Verification items for this drawing (mm, ordinates from the low corner). A direction names the side the tool comes from. Round coordinates to 2 decimals unless told otherwise and drop trailing zeros. Order: outer loops, then holes, each group sorted by start corner. A loop starts at its lowest first (then second) coordinate and runs counter-clockwise, first axis right, second up. Notation, with made-up numbers: (-0.5, -8.75) - (7.5, -8.75) arc R14 cw to (7.5, 10.25) - close; hole circle Ø5 at (80.25, 18). An arc over 180 degrees is marked (long way). Use a Markdown table: item, result. Add a question column.
(1) Section check A-A on y = 4.85. Record the boundary of the cut face in (x, z), then the cut area to 3 significant figures.
(2) Section check D-D on y = 0.65. Record the boundary of the cut face in (x, z), then the cut area to 3 significant figures.
(3) Thickness scan on line 1 along Z through (x, y) = (6, 2.55); line 2 along Y through (x, z) = (4.5, 1). Record the ranges inside material, lowest first. Write a range as [from, to].
(4) Section check C-C on z = 1. Record the boundary of the cut face in (x, y).
(5) Section check B-B on x = 3.75. Record the boundary of the cut face in (y, z), then the cut area to 3 significant figures.
(6) Gauge pin test, flat ends, axial feed: P1, Ø1.6, axis at x = 4.5, z = 1.5, coming from the +Y side; P2, Ø1, axis at x = 3, y = 1.5, coming from the +Z side; P3, Ø1.6, axis at x = 1.5, y = 4.5, coming from the +Z side. Record the tip position at first contact, or that the pin passes through.
(7) Access from +Z, -Z, +X, -X, +Y, -Y to the whole of each face (thin tool, end or side, straight path). Record for the marked faces 1, 2 and 3.
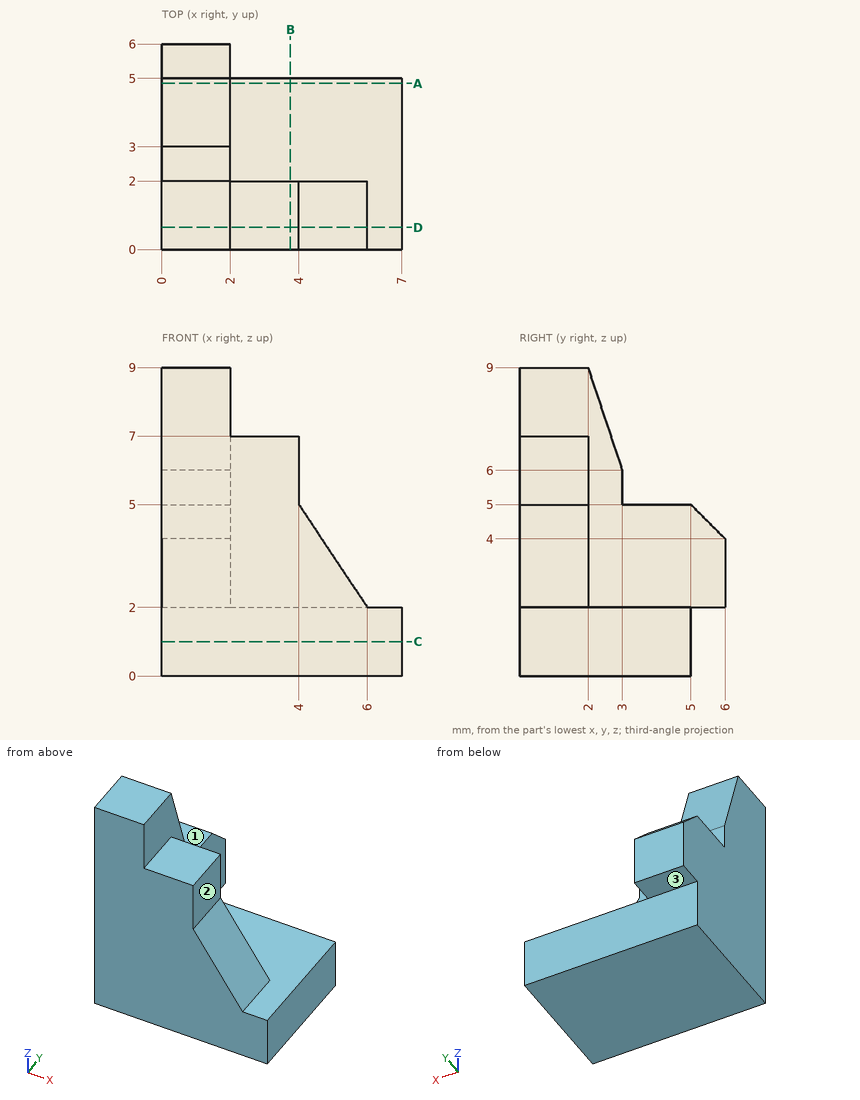
Check sheet entries:
| question | item | result |
|---|---|---|
| 1 | outline | (0, 0) - (7, 0) - (7, 2) - (2, 2) - (2, 5) - (0, 5) - close |
| 1 | area | 20.0 mm2 |
| 2 | outline | (0, 0) - (7, 0) - (7, 2) - (6, 2) - (4, 5) - (4, 7) - (2, 7) - (2, 9) - (0, 9) - close |
| 2 | area | 41.0 mm2 |
| 3 | line 1 | z = [0, 2] |
| 3 | line 2 | y = [0, 5] |
| 4 | outline | (0, 0) - (7, 0) - (7, 5) - (0, 5) - close |
| 5 | outline | (0, 0) - (5, 0) - (5, 2) - (2, 2) - (2, 7) - (0, 7) - close |
| 5 | area | 20.0 mm2 |
| 6 | P1 | stops at y = 5 |
| 6 | P2 | stops at z = 7 |
| 6 | P3 | stops at z = 5 |
| 7 | face 1 | +Z, +X, -X, +Y |
| 7 | face 2 | +Z, +X, +Y, -Y |
| 7 | face 3 | -Z, +X, -X, +Y |
